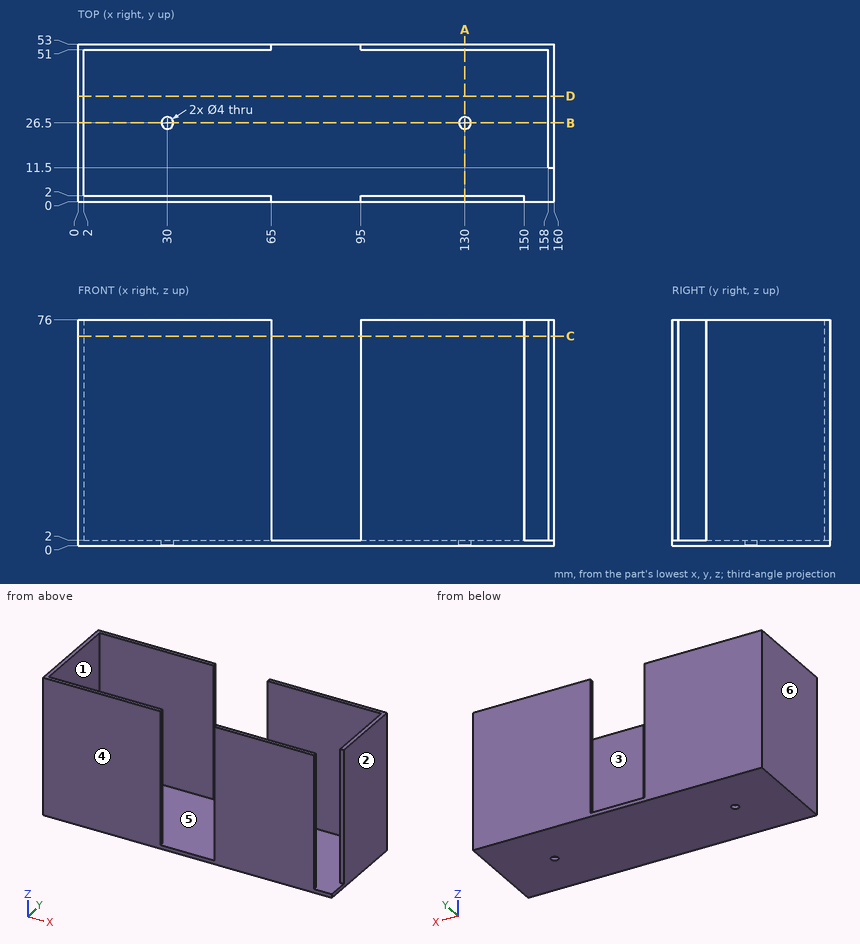
Design review of the part shown in the three views and the two pictorial views. Dimensions are in mm from the part's minimum x, y and z. A direction names the side the tool comes from. Round coordinates to 2 decimals unless told otherwise and drop trailing zeros. Write each loop counter-clockwise with the first axis right and the second up, starting at its lowest first coordinate (ties: lowest second). Pieces come first, ordered by that corner, then holes. Notation, with made-up numbers: (82.25, -39) - (132.25, -39) arc R19 cw to (132.25, -15) - close; hole circle Ø6 at (-8.5, 2). An arc over 180 degrees is marked (long way). Answer as CSV lines item,"result". Start each with the question number.
(1) Add section A-A, the plane x = 130. State the section outline as (y, z) points.
(2) For line 1 (X direction, y = 25.5, z = 54.5); line 2 (Y direction, x = 60, z = 6); line 3 (Y direction, x = 30, z = 0.55), list the stretches that pass through material, from the lowest coordinate up.
(3) Add section B-B, the plane y = 26.5. State the section outline as (x, z) points.
(4) Add section D-D, the plane y = 35.5. State the section outline as (x, z) points, plus the area to 3 significant figures.
(5) Mouldability with a two-part tool opening along Y and no side actions: class the marked faces 3, 4, 5 and 6 as +Y half, -Y half, draft (parallel to the pull), parting line (faces both ways), or undercut.
(6) Machinability: for the marked faces 1 and 2, which of the approach directions +Z, -Z, +X, -X, +Y, -Y give a long, thin tool a straight path to every point of the face, cutting with its end or side? Answer none if there is none.
(7) Add section C-C, the plane z = 70.5. State the section outline as (x, y) points, plus the area to 3 significant figures.
(8) For pin 1 (5 mm diameter, centred on x = 130, y = 26.5, fed in from +Z); pin 2 (0.6 mm diameter, centred on y = 1, z = 55, fed in from +X); pin 3 (1 mm diameter, centred on x = 159, z = 44, fed in from -Y), all flat-tipped, find the tip position at first contact; note any pin that passes through.
From the geometry:
1,outline,"(0, 0) - (24.5, 0) - (24.5, 2) - (2, 2) - (2, 76) - (0, 76) - close; (28.5, 0) - (53, 0) - (53, 76) - (51, 76) - (51, 2) - (28.5, 2) - close"
2,line 1,"x = 0 to 2, 158 to 160"
2,line 2,"y = 0 to 2, 51 to 53"
2,line 3,"y = 0 to 24.5, 28.5 to 53"
3,outline,"(0, 0) - (28, 0) - (28, 2) - (2, 2) - (2, 76) - (0, 76) - close; (32, 0) - (128, 0) - (128, 2) - (32, 2) - close; (132, 0) - (160, 0) - (160, 76) - (158, 76) - (158, 2) - (132, 2) - close"
4,outline,"(0, 0) - (160, 0) - (160, 76) - (158, 76) - (158, 2) - (2, 2) - (2, 76) - (0, 76) - close"
4,area,"616 mm²"
5,face 3,"undercut"
5,face 4,"-Y half"
5,face 5,"undercut"
5,face 6,"draft"
6,face 1,"+Z"
6,face 2,"+Z, -Z, +X, +Y, -Y"
7,outline,"(0, 0) - (65, 0) - (65, 2) - (2, 2) - (2, 51) - (65, 51) - (65, 53) - (0, 53) - close; (95, 0) - (150, 0) - (150, 2) - (95, 2) - close; (95, 51) - (158, 51) - (158, 11.5) - (160, 11.5) - (160, 53) - (95, 53) - close"
7,area,"677 mm²"
8,pin 1,"stops at z = 2"
8,pin 2,"stops at x = 150"
8,pin 3,"stops at y = 11.5"
